Autodesk Fusion 360 part; units mm, degrees
sketch "Sketch1" plane through (0, 0, 0) normal (0, 0, 1) x (1, 0, 0)
  line L0 (0, 0) -> (70.8, 0)
  line L1 (70.8, 0) -> (70.8, 15.5)
  line L2 (70.8, 15.5) -> (0, 15.5)
  line L3 (0, 15.5) -> (0, 0)
  line L4 (11.4, 15.5) -> (11.4, 0)
  line L5 (62.6, 15.5) -> (62.6, 0)
  line L6 (27.8, 15.5) -> (27.8, 4.5)
  line L7 (46.2, 15.5) -> (46.2, 4.5)
  line L8 (27.8, 4.5) -> (46.2, 4.5)
  line L9 (12.7, 15.5) -> (12.7, 4.5)
  line L10 (26.8, 15.5) -> (26.8, 4.5)
  line L11 (26.8, 4.5) -> (12.7, 4.5)
  line L12 (47.6, 15.5) -> (47.6, 4.5)
  line L13 (61.5, 15.5) -> (61.5, 4.5)
  line L14 (47.6, 4.5) -> (61.5, 4.5)
  dimension "d1" = 15.5
  dimension "d2" = 70.8
  dimension "d3" = 11.4
  dimension "d4" = 8.2
  dimension "d5" = 43
  dimension "d6" = 46.2
  dimension "d7" = 11
  dimension "d12" = 23.2
  dimension "d13" = 61.5
  dimension "d14" = 26.8
  dimension "d15" = 58.1
extrude "Extrude1" add sketch "Sketch1" along normal blind 1
extrude "Extrude2" add sketch "Sketch1" along normal blind 6 contours L0 L2 L3 L4 | L0 L1 L2 L5 | L2 L6 L7 L8
extrude "Extrude3" cut sketch "Sketch1" along normal blind 1 contours L2 L9 L10 L11 | L2 L12 L13 L14
extrude "Extrude4" add sketch "Sketch1" against normal blind 5 contours L0 L2 L3 L4 | L0 L1 L2 L5 | L2 L6 L7 L8
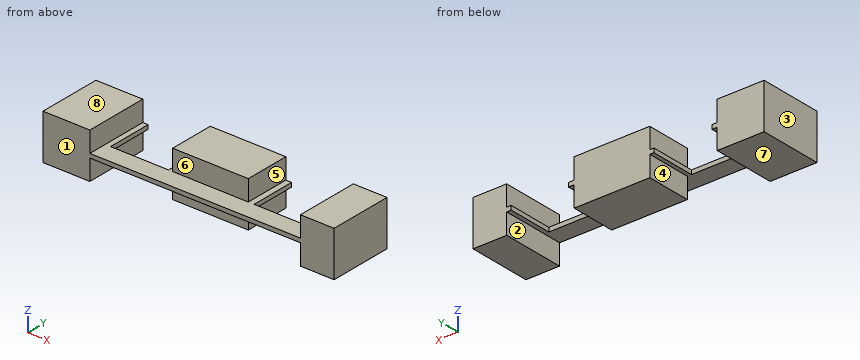
Source: CAD feature listing. Evaluate the final solid. Frame: model axes, mm. Face numbers are marked on the shaded views. A direction names the side the tool comes from. Round coordinates to 2 decimals unless told otherwise and drop trailing zeros. Loops run counter-clockwise (first coordinate to the right, second up) from the corner with the lowest first, then second, coordinate; pieces in that order, holes last.
1. Section query A-A on z = -4. Output: boundary loops of the cut face in (x, y), and give its area (3 significant figures).
2. Section query B-B on y = 7.25. Output: boundary loops of the cut face in (x, z), and give its area (3 significant figures).
3. Contact query for flat-ended pins moving along their axis: pin 1 (2 mm diameter, centred on y = 5, z = 0.5, fed in from -X); pin 2 (1.5 mm diameter, centred on x = 40, z = -3, fed in from -Y); pin 3 (1.1 mm diameter, centred on x = 53, z = 0.5, fed in from +Y). Output: stop coordinate, or through.
4. Ray query, L1, parallel to X at y = 5.75, z = -4; L2, parallel to X at y = 2.75, z = 4; L3, parallel to Z at x = 53.5, y = 3.75. Return the intervals inside material, ascending.
5. Mould query, pull axis X, two halves, no side actions, for the marked faces 1, 2 and 3. Classes: released by +X, released by -X, zero draft, split by the parting line, or undercut.
6. Section query D-D on y = 2.75. Output: boundary loops of the cut face in (x, z), and give its area (3 significant figures).
7. Access query for the marked faces 4, 5, 6, 7 and 8. Directions: +Z, -Z, +X, -X, +Y, -Y. A direction counts if a zero-diameter tool reaches every point of the face in a straight line with its end or side. Return the directions, or none.
8. Section query C-C on x = 43.5. Output: boundary loops of the cut face in (y, z), and give its area (4 significant figures).
Answers below:
1. outline: (0, 0) - (11.4, 0) - (11.4, 15.5) - (0, 15.5) - close; (27.8, 4.5) - (46.2, 4.5) - (46.2, 15.5) - (27.8, 15.5) - close; (62.6, 0) - (70.8, 0) - (70.8, 15.5) - (62.6, 15.5) - close
1. area: 506 mm2
2. outline: (0, -5) - (11.4, -5) - (11.4, 0) - (12.7, 0) - (12.7, 1) - (11.4, 1) - (11.4, 6) - (0, 6) - close; (26.8, 0) - (27.8, 0) - (27.8, -5) - (46.2, -5) - (46.2, 0) - (47.6, 0) - (47.6, 1) - (46.2, 1) - (46.2, 6) - (27.8, 6) - (27.8, 1) - (26.8, 1) - close; (61.5, 0) - (62.6, 0) - (62.6, -5) - (70.8, -5) - (70.8, 6) - (62.6, 6) - (62.6, 1) - (61.5, 1) - close
2. area: 423 mm2
3. pin 1: stops at x = 0
3. pin 2: stops at y = 4.5
3. pin 3: stops at y = 4.5
4. L1: x = 0 to 11.4, 27.8 to 46.2, 62.6 to 70.8
4. L2: x = 0 to 11.4, 62.6 to 70.8
4. L3: z = 0 to 1
5. face 1: zero draft
5. face 2: undercut
5. face 3: released by -X
6. outline: (0, -5) - (11.4, -5) - (11.4, 0) - (62.6, 0) - (62.6, -5) - (70.8, -5) - (70.8, 6) - (62.6, 6) - (62.6, 1) - (11.4, 1) - (11.4, 6) - (0, 6) - close
6. area: 267 mm2
7. face 4: -Z, +Y, -Y
7. face 5: +Z, +Y, -Y
7. face 6: +Z, -Y
7. face 7: -Z, +X, -X, +Y, -Y
7. face 8: +Z, +X, -X, +Y, -Y
8. outline: (0, 0) - (4.5, 0) - (4.5, -5) - (15.5, -5) - (15.5, 6) - (4.5, 6) - (4.5, 1) - (0, 1) - close
8. area: 125.5 mm2
